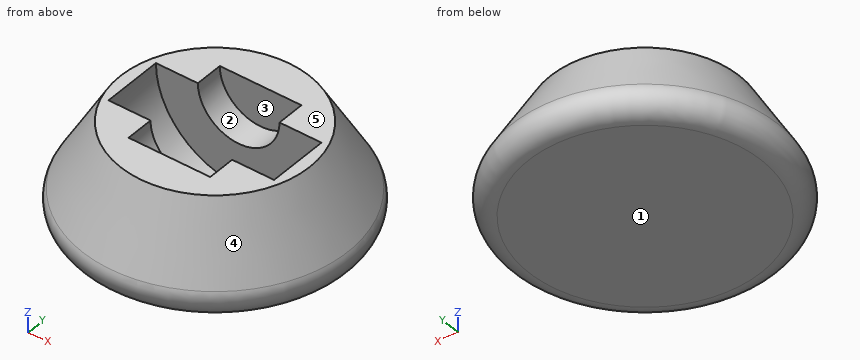
from build123d import *

# Parameters (mm, degrees)
F4_DEPTH = 8
F5_R     = 5
F6_R     = 10.7775
F7_DEPTH = 15.4


with BuildPart() as f2:
    # F1 (on Front) → F2 (revolve)
    with BuildSketch(Plane.XZ):
        Polygon((-39.4337567297, 0), (0, 0), (0, 25), (-25, 25), align=None)
    revolve(axis=Axis((0, 0, 12.5), (0, 0, -1)))

    # F3 (on Front) → F4 (cut, symmetric)
    with BuildSketch(Plane.XZ):
        with BuildLine():
            Line((21.855, 25), (0, 25))
            Line((0, 25), (0, 3.145))
            ThreePointArc((0, 3.145), (15.4538187028, 9.5461812972), (21.855, 25))
        make_face()
        with BuildLine():
            Line((0, 3.145), (0, 25))
            Line((0, 25), (-21.855, 25))
            ThreePointArc((-21.855, 25), (-15.4538187028, 9.5461812972), (0, 3.145))
        make_face()
    extrude(amount=F4_DEPTH, both=True, mode=Mode.SUBTRACT)

    # F5
    f5_edges = [f2.edges().sort_by_distance(p)[0] for p in [
        (39.433757, 0, 0),
    ]]
    fillet(f5_edges, radius=F5_R)

    # F6 (on Front) → F7 (cut, symmetric)
    with BuildSketch(Plane.XZ):
        with Locations((0, 25)):
            Circle(F6_R)
    extrude(amount=F7_DEPTH, both=True, mode=Mode.SUBTRACT)


solid = f2.part
For this review, take the finished solid that the model builds, in its own axes (mm). Face numbers are marked on the shaded views. A direction names the side the tool comes from. Round coordinates to 2 decimals unless told otherwise and drop trailing zeros. Loops run counter-clockwise (first coordinate to the right, second up) from the corner with the lowest first, then second, coordinate; pieces in that order, holes last. Notation, with made-up numbers: (79.25, 16.5) - (95.25, 16.5) arc R18 ccw to (95.25, 44.5) - close; hole circle Ø9 at (41.5, 73). An arc over 180 degrees is marked (long way). Use one line per item in the form item = value.
Item 1: Tool access review of the marked faces 1 and 2: name each direction out of +Z, -Z, +X, -X, +Y, -Y from which nothing blocks a thin tool from reaching the whole face with its end or side.
Answers:
face_1 = -Z, +X, -X, +Y, -Y
face_2 = +Z
Item 2: Consider section D-D on z = 2. Write out the cut boundary in (x, y).
Answers:
outline = circle Ø69.55 at (0, 0)
Item 3: Consider section C-C on z = 15.25. Write out the cut boundary in (x, y), then the cut area to 3 significant figures.
Answers:
outline = circle Ø61.26 at (0, 0); hole (-19.56, -8) - (-4.59, -8) - (-4.59, -15.4) - (4.59, -15.4) - (4.59, -8) - (19.56, -8) - (19.56, 8) - (4.59, 8) - (4.59, 15.4) - (-4.59, 15.4) - (-4.59, 8) - (-19.56, 8) - close
area = 2,190 mm^2
Item 4: Mouldability with a two-part tool opening along Y and no side actions: class the marked faces 3, 4 and 5 as +Y half, -Y half, draft (parallel to the pull), parting line (faces both ways), or undercut.
Answers:
face_3 = undercut
face_4 = parting line
face_5 = draft
Item 5: Consider section A-A on z = 19.75. Write out the cut boundary in (x, y).
Answers:
outline = circle Ø56.06 at (0, 0); hole (-21.22, -8) - (-9.41, -8) - (-9.41, -15.4) - (9.41, -15.4) - (9.41, -8) - (21.22, -8) - (21.22, 8) - (9.41, 8) - (9.41, 15.4) - (-9.41, 15.4) - (-9.41, 8) - (-21.22, 8) - close
Item 6: Consider section B-B on y = 0. Write out the cut boundary in (x, z) (1 decimal), then the cut area to 3 significant figures.
Answers:
outline = (-35.1, 7.5) arc R5 ccw to (-30.8, 0) - (30.8, 0) arc R5 ccw to (35.1, 7.5) - (25, 25) - (21.9, 25) arc R21.9 cw to (-21.9, 25) - (-25, 25) - close
area = 826 mm^2
Item 7: Clearance check with flat-ended pins moving along their axes: P1, Ø5, axis at x = -10.5, z = 4, coming from the -Y side; P2, Ø12, axis at y = -6, z = 22.5, coming from the +X side; P3, Ø4, axis at y = 5.5, z = 16, coming from the -X side. State where each tip first meets the part, or that it passes through.
Answers:
P1 = -34.84
P2 = 29.46
P3 = -30.91
Item 8: For line 1 (Z direction, x = 0.5, y = 12); line 2 (Y direction, x = -6.5, z = 17); line 3 (Y direction, x = 6, z = 14), list the stretches that pass through material, from the lowest coordinate up.
Answers:
line_1 = 0 to 14.23
line_2 = -28.9 to -15.4, 15.4 to 28.9
line_3 = -30.77 to -8, 8 to 30.77
